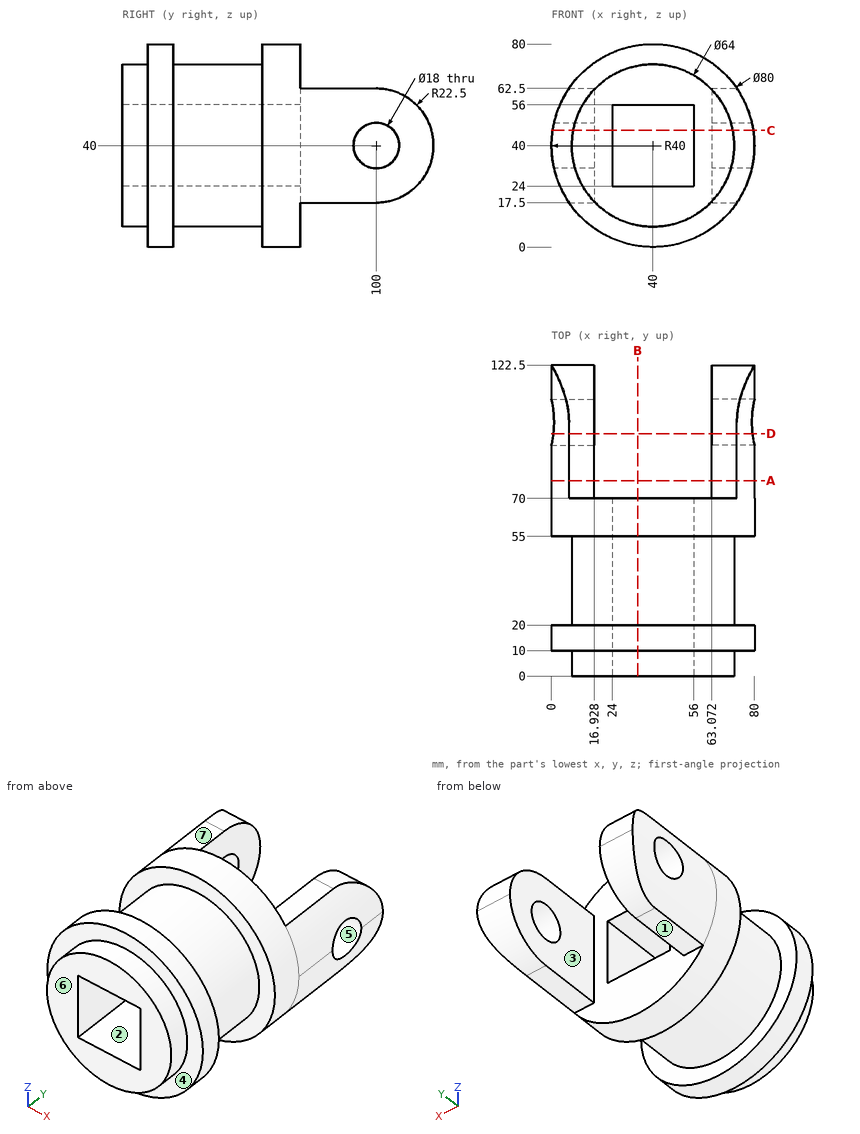
The drawing under review shows one solid part. Ordinate dimensions are in mm from its lowest x, y, z. A direction names the side the tool comes from. Give positions to 0.01 mm unless a question says otherwise; leave off trailing zeros. Order: outer loops, then holes, each group sorted by start corner. A loop starts at its lowest first (then second) coordinate and runs counter-clockwise, first axis right, second up. Notation, with made-up numbers: M 33.5,63.5 L 76.5,63.5 A29 ccw 76.5,86.5 Z; hole C 84,-6.5 d5. An arc over 180 degrees is marked long. One line per question, with ' | ' between items. Start each with the question number.
Q1. For pin 1 Ø5 at (x, y) = (69.5, 89.5) entering from -Z; pin 2 Ø9.5 at (y, z) = (28.5, 41) entering from -X; pin 3 Ø24 at (x, z) = (54, 26) entering from -Y; pin 4 Ø9.5 at (x, y) = (37.5, 30.5) entering from +Z, all flat-tipped, find the tip position at first contact; note any pin that passes through.
Q2. We need section D-D (y = 95.5). Write out the cut boundary in (x, z).
Q3. The part is to be moulded in two halves that separate along Y. For the marked faces 5, 6 and 7, say which applies: +Y half, -Y half, draft (parallel to the pull), parting line (faces both ways), or undercut.
Q4. For L1, parallel to Y at x = 76.25, z = 40; L2, parallel to Y at x = 70, z = 40; L3, parallel to Z at x = 9, y = 100, list the stretches that pass through material, from the lowest coordinate up. Write a range as [from, to].
Q5. We need section B-B (x = 34). Write out the cut boundary in (y, z), plus the area to 3 significant figures.
Q6. Machinability: for the marked faces 1, 2, 3 and 4, which of the approach directions +Z, -Z, +X, -X, +Y, -Y give a long, thin tool a straight path to every point of the face, cutting with its end or side? Answer none if there is none.
Q7. We need section C-C (z = 46). State how many separate pieces and enclosed holes the cut face has, plus the area to 3 significant figures.
Q8. We need section A-A (y = 77). Write out the cut boundary in (x, z), plus the area to 3 significant figures.
Returned:
1) pin 1: z = 17.5 | pin 2: x = 8 | pin 3: y = 0 | pin 4: z = 72
2) outline: M 0.77,32.21 A40 ccw 6.93,17.5 L 16.93,17.5 L 16.93,32.21 Z; M 0.77,47.79 L 16.93,47.79 L 16.93,62.5 L 6.93,62.5 A40 ccw Z; M 63.07,17.5 L 73.07,17.5 A40 ccw 79.23,32.21 L 63.07,32.21 Z; M 63.07,47.79 L 79.23,47.79 A40 ccw 73.07,62.5 L 63.07,62.5 Z
3) face 5: undercut | face 6: -Y half | face 7: draft
4) L1: [10, 20], [55, 91], [109, 122.5] | L2: [0, 91], [109, 122.5] | L3: [17.5, 31], [49, 62.5]
5) outline: M 0,8.57 L 10,8.57 L 10,0.45 L 20,0.45 L 20,8.57 L 55,8.57 L 55,0.45 L 70,0.45 L 70,24 L 0,24 Z; M 0,56 L 70,56 L 70,79.55 L 55,79.55 L 55,71.43 L 20,71.43 L 20,79.55 L 10,79.55 L 10,71.43 L 0,71.43 Z | area: 2,570 mm2
6) face 1: -Z, +X, -X, +Y | face 2: +Y, -Y | face 3: +Z, -Z, +Y | face 4: -Y
7) separate pieces: 4 | enclosed holes: 0 | area: 3,830 mm2
8) outline: M 6.93,17.5 L 16.93,17.5 L 16.93,62.5 L 6.93,62.5 A40 ccw Z; M 63.07,17.5 L 73.07,17.5 A40 ccw 73.07,62.5 L 63.07,62.5 Z | area: 1,320 mm2
